from build123d import *

# Parameters (mm, degrees)
SKETCH_W        = 76.2
SKETCH_H        = 76.2
PAD_DEPTH       = 8
SKETCH002_R     = 2.25
POCKET001_DEPTH = 10.001
SKETCH003_R     = 23
POCKET002_DEPTH = 6
SKETCH004_R     = 2.55
PAD001_DEPTH    = 7
SKETCH006_R     = 30.165
POCKET_DEPTH    = 1.4
CHAMFER_SIZE    = 1
FILLET_R        = 4.5
FILLET001_R     = 1.25
FILLET002_R     = 2
SKETCH005_R     = 1.5
POCKET003_DEPTH = 30


with BuildPart() as part:
    # Sketch → Pad (new body)
    with BuildSketch(Plane.XY):
        with Locations((38.1, 38.1)):
            Rectangle(SKETCH_W, SKETCH_H)
    extrude(amount=PAD_DEPTH)

    # Sketch002 → Pocket001 (cut, through all)
    with BuildSketch(Plane.XY.offset(10)):
        with Locations((8, 8)):
            Circle(SKETCH002_R)
        with Locations((8, 68.2)):
            Circle(SKETCH002_R)
        with Locations((68.2, 68.2)):
            Circle(SKETCH002_R)
        with Locations((68.2, 8)):
            Circle(SKETCH002_R)
    extrude(amount=-POCKET001_DEPTH, mode=Mode.SUBTRACT)

    # Sketch003 (on Face5 of Pocket001) → Pocket002 (cut)
    with BuildSketch(Plane.XY.offset(8)):
        with Locations((38.1, 38.1)):
            Circle(SKETCH003_R)
    extrude(amount=-POCKET002_DEPTH, mode=Mode.SUBTRACT)

    # Sketch004 (on Face2 of Pocket002) → Pad001 (join)
    with BuildSketch(Plane(origin=(0, 0, 0), x_dir=(0, -1, 0), z_dir=(-1, 0, 0))):
        with Locations((-38.1, 4)):
            Circle(SKETCH004_R)
    extrude(amount=PAD001_DEPTH)

    # Sketch006 (on Face5 of Pad001) → Pocket (cut)
    with BuildSketch(Plane.XY.offset(8)):
        with Locations((38.1, 38.1)):
            Circle(SKETCH006_R)
    extrude(amount=-POCKET_DEPTH, mode=Mode.SUBTRACT)

    # Chamfer
    chamfer_edges = [part.edges().sort_by_distance(p)[0] for p in [
        (-7, 40.65, 4),
    ]]
    chamfer(chamfer_edges, length=CHAMFER_SIZE)

    # Fillet
    fillet_edges = [part.edges().sort_by_distance(p)[0] for p in [
        (15.1, 38.1, 2),
    ]]
    fillet(fillet_edges, radius=FILLET_R)

    # Fillet001
    fillet001_edges = [part.edges().sort_by_distance(p)[0] for p in [
        (7.935, 38.1, 6.6),
    ]]
    fillet(fillet001_edges, radius=FILLET001_R)

    # Fillet002
    fillet002_edges = [part.edges().sort_by_distance(p)[0] for p in [
        (0, 40.65, 4),
    ]]
    fillet(fillet002_edges, radius=FILLET002_R)

    # Sketch005 (on Face13 of Pad001) → Pocket003 (cut)
    with BuildSketch(Plane(origin=(-7, 0, 0), x_dir=(0, -1, 0), z_dir=(-1, 0, 0))):
        with Locations((-38.1, 4)):
            Circle(SKETCH005_R)
    extrude(amount=-POCKET003_DEPTH, mode=Mode.SUBTRACT)


solid = part.part
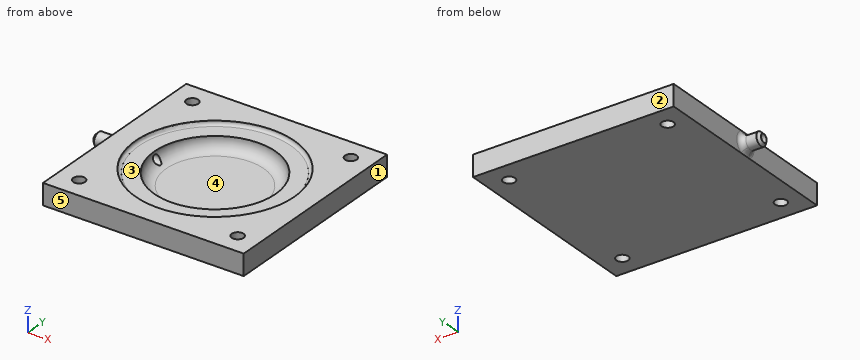
The model under review builds one solid part; all positions refer to its coordinate system, in mm. Face numbers are marked on the shaded views. A direction names the side the tool comes from. Coordinates: 2 decimals unless noted, no trailing zeros. Loops run counter-clockwise (first coordinate to the right, second up) from the corner with the lowest first, then second, coordinate; pieces in that order, holes last.
(1) Draft analysis for pull direction Y (two halves, no side actions). For the marked faces 1, 2 and 3, state which applies: +Y half, -Y half, draft (parallel to the pull), parting line (faces both ways), or undercut.
Determined:
face 1: draft
face 2: +Y half
face 3: undercut
(2) Insertion check: P1, Ø6, axis at x = 68.2, y = 8, coming from the +Z side; P2, Ø1, axis at y = 68.5, z = 1, coming from the -X side; P3, Ø17.5, axis at x = 37, y = 48.5, coming from the +Z side. Each pin has a flat end and moves straight along its axis. Give the tip position at first contact, or say it passes through.
Determined:
P1: stops at z = 8
P2: stops at x = 0
P3: stops at z = 2.06
(3) Consider section B-B, the plane z = 4. Give the boundary of the cut face in (x, y), plus the area to 3 significant figures.
Determined:
outline: (-7, 36.55) - (-6, 35.55) - (-2, 35.55) arc R2 cw to (0, 33.55) - (0, 0) - (76.2, 0) - (76.2, 76.2) - (0, 76.2) - (0, 42.65) arc R2 cw to (-2, 40.65) - (-6, 40.65) - (-7, 39.65) - (-7, 39.6) - (15.91, 39.6) arc R22.24 cw (long way) to (15.91, 36.6) - (-7, 36.6) - close; hole circle Ø4.5 at (8, 8); hole circle Ø4.5 at (8, 68.2); hole circle Ø4.5 at (68.2, 8); hole circle Ø4.5 at (68.2, 68.2)
area: 4,160 mm2
(4) Tool access review of the marked faces 4 and 5: name each direction out of +Z, -Z, +X, -X, +Y, -Y from which nothing blocks a thin tool from reaching the whole face with its end or side.
Determined:
face 4: +Z
face 5: +Z, -Z, +X, -X, -Y
(5) Wall thickness on L1, parallel to Y at x = 68.2, z = 3; L2, parallel to Y at x = 38.1, z = 7.9 (3 decimals); L3, parallel to Z at x = 54, y = 28: over which ranges is each line inside the solid? List them lowest first.
Determined:
L1: y = 0 to 5.75, 10.25 to 65.95, 70.45 to 76.2
L2: y = 0 to 7.935, 68.265 to 76.2
L3: z = 0 to 2.01
(6) Consider section A-A, the plane x = 38.1. Give the boundary of the cut face in (y, z) (3 decimals), plus the area to 3 significant figures.
Determined:
outline: (0, 0) - (76.2, 0) - (76.2, 8) - (68.265, 8) - (68.265, 7.85) arc R1.25 cw to (67.015, 6.6) - (61.1, 6.6) - (61.1, 6.5) arc R4.5 cw to (56.6, 2) - (19.6, 2) arc R4.5 cw to (15.1, 6.5) - (15.1, 6.6) - (9.185, 6.6) arc R1.25 cw to (7.935, 7.85) - (7.935, 8) - (0, 8) - close
area: 323 mm2
